Geometry: see drawing. Coordinates: mm, zero at the bounding-box minimum. A direction names the side the tool comes from. Round coordinates to 2 decimals unless told otherwise and drop trailing zeros. Write each loop counter-clockwise with the first axis right and the second up, starting at its lowest first coordinate (ties: lowest second). Pieces come first, ordered by that corner, then holes. Notation, with made-up numbers: M 16.25,3 L 62.25,3 A29 cw 62.25,37 Z; hole C 27.5,14 d6. An arc over 180 degrees is marked long. Use a Markdown table: item, result.
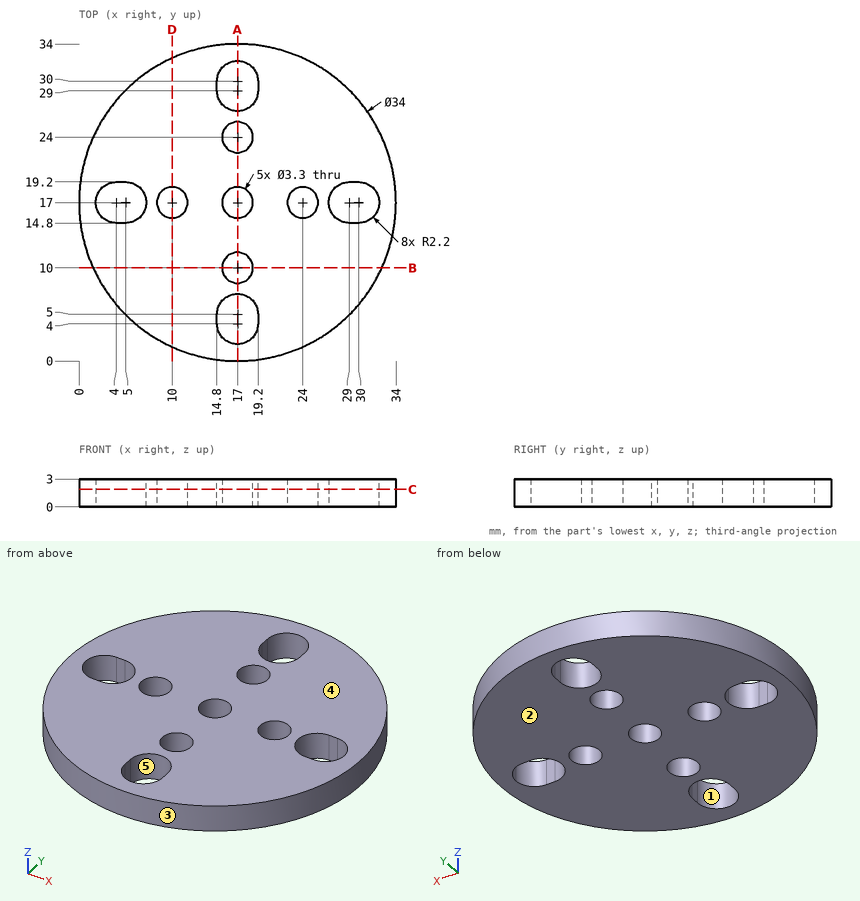
Q1. Section B-B on y = 10. Return loops of the section in (x, z), plus the area to 3 significant figures.
Results are:
| item | result |
|---|---|
| outline | M 1.51,0 L 15.35,0 L 15.35,3 L 1.51,3 Z; M 18.65,0 L 32.49,0 L 32.49,3 L 18.65,3 Z |
| area | 83.1 mm^2 |
Q2. Line query: L1, parallel to Y at x = 17, z = 1.8; L2, parallel to Y at x = 16.5, z = 1.55; L3, parallel to X at y = 18, z = 1.4. Output: solid intervals per line, ascending.
Results are:
| item | result |
|---|---|
| L1 | 0 to 1.8, 7.2 to 8.35, 11.65 to 15.35, 18.65 to 22.35, 25.65 to 26.8, 32.2 to 34 |
| L2 | 0.01 to 1.86, 7.14 to 8.43, 11.57 to 15.43, 18.57 to 22.43, 25.57 to 26.86, 32.14 to 33.99 |
| L3 | 0.03 to 2.04, 6.96 to 8.69, 11.31 to 15.69, 18.31 to 22.69, 25.31 to 27.04, 31.96 to 33.97 |
Q3. Reachability of the marked faces 4 and 5 from +Z, -Z, +X, -X, +Y, -Y: full face, straight path, thin tool, end or side. Return the list, or none.
Results are:
| item | result |
|---|---|
| face 4 | +Z, +X, -X, +Y, -Y |
| face 5 | +Z, -Z |
Q4. Section A-A on x = 17. Return loops of the section in (y, z), plus the area to 3 significant figures.
Results are:
| item | result |
|---|---|
| outline | M 0,0 L 1.8,0 L 1.8,3 L 0,3 Z; M 7.2,0 L 8.35,0 L 8.35,3 L 7.2,3 Z; M 11.65,0 L 15.35,0 L 15.35,3 L 11.65,3 Z; M 18.65,0 L 22.35,0 L 22.35,3 L 18.65,3 Z; M 25.65,0 L 26.8,0 L 26.8,3 L 25.65,3 Z; M 32.2,0 L 34,0 L 34,3 L 32.2,3 Z |
| area | 39.9 mm^2 |
Q5. First-contact query: pin 1 Ø0.8 at (x, z) = (29.5, 1.5) entering from +Y; pin 2 Ø4 at (x, y) = (17, 17) entering from +Z; pin 3 Ø0.5 at (y, z) = (4.5, 1.5) entering from -X; pin 4 Ø0.8 at (y, z) = (4.5, 2) entering from +X. Flat tips, straight axial feed; report the tip coordinate or a pass-through.
Results are:
| item | result |
|---|---|
| pin 1 | y = 28.94 |
| pin 2 | z = 3 |
| pin 3 | x = 5.21 |
| pin 4 | x = 28.94 |
Q6. Mould query, pull axis Y, two halves, no side actions, for the marked faces 1, 2 and 3. Classes: +Y half, -Y half, draft (parallel to the pull), parting line (faces both ways), or undercut.
Results are:
| item | result |
|---|---|
| face 1 | undercut |
| face 2 | draft |
| face 3 | parting line |
Q7. Section C-C on z = 1.9. Give the number of separate pieces and of enclosed holes in the cut face, plus the area to 3 significant figures.
Results are:
| item | result |
|---|---|
| separate pieces | 1 |
| enclosed holes | 9 |
| area | 787 mm^2 |
